Here's how the part is built. I have some questions about the finished solid (model axes, mm). A direction names the side the tool comes from. Coordinates: 2 decimals unless noted, no trailing zeros. Loops run counter-clockwise (first coordinate to the right, second up) from the corner with the lowest first, then second, coordinate; pieces in that order, holes last. Notation, with made-up numbers: (45.25, -33) -> (78.25, -33) arc R6 cw to (78.25, -25) -> close; hole circle Ø2 at (47, 9.25). An arc over 180 degrees is marked (long way). Answer as a JSON object with one key per item and string values. Group by question number.
Q1. I'm going to push flat-ended pins straight in: pin 1 (3 mm diameter, centred on x = 24.45, y = 28.61, fed in from +Z); pin 2 (4 mm diameter, centred on x = -18, y = -42, fed in from -Z); pin 3 (5 mm diameter, centred on x = 27, z = 6, fed in from -Y) (3 decimals); pin 4 (1.5 mm diameter, centred on x = 0, z = 16.5, fed in from -Y) (3 decimals). Where does each tip first touch, or does it pass through?
Q2. On a 3-axis mill with a long thin cutter (end or side, diameter ignored), from which of +Z, -Z, +X, -X, +Y, -Y can I reach the whole of each face in a straight line? I mean faces 1 (the flat face through (-19.45, 60, 10)), 2 (the flat face through (24, -63.225, 9)), 3 (the flat face through (-19.45, 0, 17)). Say none if no direction works.
Q3. I want a section at B-B on y = 28.61. Write out the boundary of the cut face in (x, z), then the cut area to 3 significant figures.
Q4. I want a section at D-D on x = -21. Write out the boundary of the cut face in (y, z) (3 decimals).
Q5. Thinking about a two-plate mould opening in X: for faces 4 (the flat face through (0, -45.605, 17)), 5 (the flat face through (24, -64, 0)), 6 (the flat face through (29.45, 0, 17)), which applies, released by +X, released by -X, zero draft, split by the parting line, or undercut?
Q6. I want a section at A-A on x = -9. Write out the boundary of the cut face in (y, z) (3 decimals).
Q7. I want a section at C-C on z = 4.5. Write out the boundary of the cut face in (x, y) (3 decimals), then the cut area to 3 significant figures.
Q8. I need wall thicknesses on line 1 (X direction, y = -28.61, z = 16.2); line 2 (Y direction, x = 24.45, z = 1.2) (3 decimals); line 3 (Y direction, x = 6.5, z = 19) (3 decimals). Which ranges of each line are inside material? Lowest first, please.
```python
from build123d import *

# Parameters (mm, degrees)
ESQUISSE1_W                = 10
ESQUISSE1_H                = 146.45
BOSS_EXTRU_3_DEPTH         = 3
ESQUISSE3_W                = 10
ESQUISSE3_H                = 126.45
BOSS_EXTRU_4_DEPTH         = 17
ESQUISSE4_R                = 1.84
ENL_V_MAT_EXTRU_1_DEPTH    = 17
ESQUISSE5_R                = 1.84
ENL_V_MAT_EXTRU_2_DEPTH    = 82.419918478
ESQUISSE6_W                = 15
ESQUISSE6_H                = 111.45
ENL_V_MAT_EXTRU_3_DEPTH    = 77.563049998
CONG_1_R                   = 5
CONG_2_R                   = 5
R_P_TITION_LIN_AIRE1_COUNT = 2
R_P_TITION_LIN_AIRE1_PITCH = 48.9
ESQUISSE7_W                = 58.9
ESQUISSE7_H                = 10
BOSS_EXTRU_5_DEPTH         = 5
CONG_4_R                   = 2
ESQUISSE8_W                = 58.9
ESQUISSE8_H                = 10
BOSS_EXTRU_6_DEPTH         = 5
CONG_5_R                   = 2


with BuildPart() as part:
    # Esquisse1 → Boss.-Extru.3 (new body)
    with BuildSketch(Plane.XY):
        with Locations((-24.45, 0)):
            Rectangle(ESQUISSE1_W, ESQUISSE1_H)
    extrude(amount=BOSS_EXTRU_3_DEPTH)

    # Esquisse3 → Boss.-Extru.4 (add)
    with BuildSketch(Plane.XY.offset(3)):
        with Locations((-24.45, 0)):
            Rectangle(ESQUISSE3_W, ESQUISSE3_H)
    extrude(amount=BOSS_EXTRU_4_DEPTH)

    # Esquisse4 → Enl_v. mat.-Extru.1 (cut)
    with BuildSketch(Plane.XY.offset(3)):
        with Locations((-24.45, -68.225)):
            Circle(ESQUISSE4_R)
    enl_v_mat_extru_1 = extrude(amount=-ENL_V_MAT_EXTRU_1_DEPTH, mode=Mode.SUBTRACT)

    # Sym_trie1: Enl_v. mat.-Extru.1 across plane
    add(enl_v_mat_extru_1.mirror(Plane.ZX), mode=Mode.SUBTRACT)

    # Esquisse5 → Enl_v. mat.-Extru.2 (cut, through all)
    with BuildSketch(Plane.XY.offset(20)):
        with Locations((-24.45, 28.61)):
            Circle(ESQUISSE5_R)
    enl_v_mat_extru_2 = extrude(amount=-ENL_V_MAT_EXTRU_2_DEPTH, mode=Mode.SUBTRACT)

    # Sym_trie2: Enl_v. mat.-Extru.2 across plane
    add(enl_v_mat_extru_2.mirror(Plane.ZX), mode=Mode.SUBTRACT)

    # Esquisse6 → Enl_v. mat.-Extru.3 (cut, through all)
    with BuildSketch(Plane.ZY.offset(29.45)):
        with Locations((7.5, 0)):
            Rectangle(ESQUISSE6_W, ESQUISSE6_H)
    extrude(amount=-ENL_V_MAT_EXTRU_3_DEPTH, mode=Mode.SUBTRACT)

    # Cong_1
    cong_1_edges = [part.edges().sort_by_distance(p)[0] for p in [
        (-24.45, -63.225, 20),
        (-24.45, 63.225, 20),
    ]]
    fillet(cong_1_edges, radius=CONG_1_R)

    # Cong_2
    cong_2_edges = [part.edges().sort_by_distance(p)[0] for p in [
        (-24.45, 55.725, 15),
        (-24.45, -55.725, 15),
    ]]
    fillet(cong_2_edges, radius=CONG_2_R)


with BuildPart() as r_p_tition_lin_aire1_1:
    # R_p_tition lin_aire1: pattern copy
    add(part.part.moved(Location(Vector(1, 0, 0) * (1 * R_P_TITION_LIN_AIRE1_PITCH))))


with BuildPart() as part_1:
    add(part.part)

    add(r_p_tition_lin_aire1_1.part)  # Boss.-Extru.5 merges R_p_tition lin_aire1_1
    # Esquisse7 → Boss.-Extru.5 (add)
    with BuildSketch(Plane(origin=(0, 0, 15), x_dir=(-1, 0, 0), z_dir=(0, 0, -1))):
        with Locations((0, 40.605950242)):
            Rectangle(ESQUISSE7_W, ESQUISSE7_H)
    extrude(amount=-BOSS_EXTRU_5_DEPTH)

    # Cong_4
    cong_4_edges = [part_1.edges().sort_by_distance(p)[0] for p in [
        (-19.45, 45.605950242, 17.5),
        (-19.45, 35.605950242, 17.5),
        (19.45, 35.605950242, 17.5),
        (19.45, 45.605950242, 17.5),
    ]]
    fillet(cong_4_edges, radius=CONG_4_R)

    # Esquisse8 → Boss.-Extru.6 (add)
    with BuildSketch(Plane(origin=(0, 0, 15), x_dir=(-1, 0, 0), z_dir=(0, 0, -1))):
        with Locations((0, -40.605)):
            Rectangle(ESQUISSE8_W, ESQUISSE8_H)
    extrude(amount=-BOSS_EXTRU_6_DEPTH)

    # Cong_5
    cong_5_edges = [part_1.edges().sort_by_distance(p)[0] for p in [
        (19.45, -45.605, 17.5),
        (19.45, -35.605, 17.5),
        (-19.45, -35.605, 17.5),
        (-19.45, -45.605, 17.5),
    ]]
    fillet(cong_5_edges, radius=CONG_5_R)


solid = part_1.part
```
Result set:
{
 "1": {"pin 1": "passes through", "pin 2": "stops at z = 15", "pin 3": "stops at y = -63.225", "pin 4": "stops at y = -45.605"},
 "2": {"face 1": "+Z, -Z, +Y", "face 2": "+Z, +X, -X, -Y", "face 3": "+Z, -Z"},
 "3": {"outline": "(-29.45, 15) -> (-26.29, 15) -> (-26.29, 20) -> (-29.45, 20) -> close; (-22.61, 15) -> (-19.45, 15) -> (-19.45, 20) -> (-22.61, 20) -> close; (19.45, 15) -> (22.61, 15) -> (22.61, 20) -> (19.45, 20) -> close; (26.29, 15) -> (29.45, 15) -> (29.45, 20) -> (26.29, 20) -> close", "area": "63.2 mm²"},
 "4": {"outline": "(-73.225, 0) -> (-55.725, 0) -> (-55.725, 10) arc R5 cw to (-50.725, 15) -> (50.725, 15) arc R5 cw to (55.725, 10) -> (55.725, 0) -> (73.225, 0) -> (73.225, 3) -> (63.225, 3) -> (63.225, 15) arc R5 ccw to (58.225, 20) -> (-58.225, 20) arc R5 ccw to (-63.225, 15) -> (-63.225, 3) -> (-73.225, 3) -> close"},
 "5": {"face 4": "undercut", "face 5": "zero draft", "face 6": "released by +X"},
 "6": {"outline": "(-45.605, 15) -> (-35.605, 15) -> (-35.605, 20) -> (-45.605, 20) -> close; (35.606, 15) -> (45.606, 15) -> (45.606, 20) -> (35.606, 20) -> close"},
 "7": {"outline": "(-29.45, -63.225) -> (-19.45, -63.225) -> (-19.45, -55.725) -> (-29.45, -55.725) -> close; (-29.45, 55.725) -> (-19.45, 55.725) -> (-19.45, 63.225) -> (-29.45, 63.225) -> close; (19.45, -63.225) -> (29.45, -63.225) -> (29.45, -55.725) -> (19.45, -55.725) -> close; (19.45, 55.725) -> (29.45, 55.725) -> (29.45, 63.225) -> (19.45, 63.225) -> close", "area": "300 mm²"},
 "8": {"line 1": "x = -29.45 to -26.29, -22.61 to -19.45, 19.45 to 22.61, 26.29 to 29.45", "line 2": "y = -73.225 to -70.065, -66.385 to -55.725, 55.725 to 66.385, 70.065 to 73.225", "line 3": "y = -45.605 to -35.605, 35.606 to 45.606"}
}
